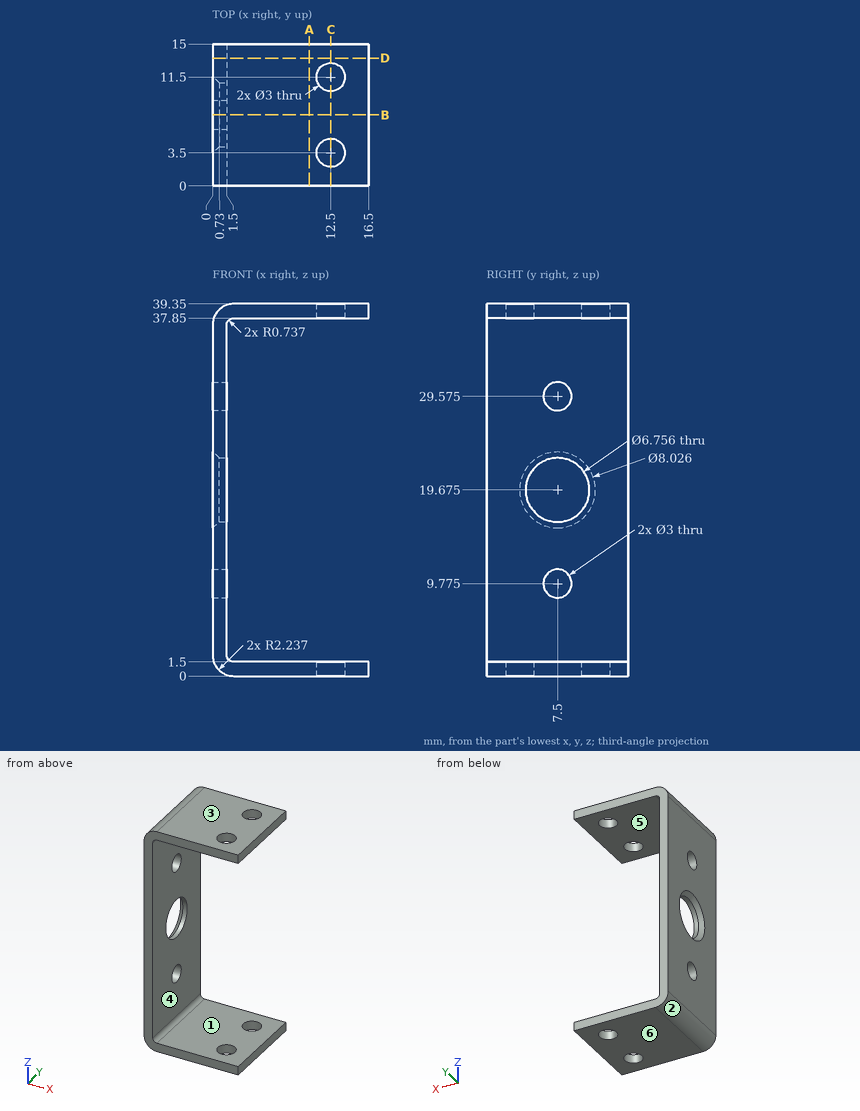
Design review of the part shown in the three views and the two pictorial views. Dimensions are in mm from the part's minimum x, y and z. A direction names the side the tool comes from. Round coordinates to 2 decimals unless told otherwise and drop trailing zeros. Write each loop counter-clockwise with the first axis right and the second up, starting at its lowest first coordinate (ties: lowest second). Pieces come first, ordered by that corner, then holes.
Item 1: Consider section C-C on x = 12.5. Give the boundary of the cut face in (y, z).
Item 2: For pin 1 Ø6 at (y, z) = (9.5, 13.5) entering from +X, flat-tipped, find the tip position at first contact; note if it passes through.
Item 3: Wall thickness on L1, parallel to Y at x = 12.5, z = 39; L2, parallel to Z at x = 4.25, y = 2: over which ranges is each line inside the solid? List them lowest first.
Item 4: Consider section D-D on y = 13.5. Give the boundary of the cut face in (x, z), and give its area (3 significant figures).
Item 5: For the marked faces 1 and 2, list the 3-axis set-ups (+Z, -Z, +X, -X, +Y, -Y) from which the entire face can be reached by the end or side of a thin tool; tool diameter is ignored.
Item 6: Consider section A-A on x = 10.25. Give the boundary of the cut face in (y, z).
Item 7: Draft analysis for pull direction Z (two halves, no side actions). For the marked faces 3, 4, 5 and 6, state which applies: released by +Z, released by -Z, zero draft, split by the parting line, or undercut.
Item 8: Consider section B-B on y = 7.5. Count the separate pieces of the cut face and the enclosed holes in it.
Check values:
1. outline: (0, 0) - (2, 0) - (2, 1.5) - (0, 1.5) - close; (0, 37.85) - (2, 37.85) - (2, 39.35) - (0, 39.35) - close; (5, 0) - (10, 0) - (10, 1.5) - (5, 1.5) - close; (5, 37.85) - (10, 37.85) - (10, 39.35) - (5, 39.35) - close; (13, 0) - (15, 0) - (15, 1.5) - (13, 1.5) - close; (13, 37.85) - (15, 37.85) - (15, 39.35) - (13, 39.35) - close
2. pin 1: stops at x = 1.5
3. L1: y = 0 to 2, 5 to 10, 13 to 15
3. L2: z = 0 to 1.5, 37.85 to 39.35
4. outline: (0, 2.24) arc R2.24 ccw to (2.24, 0) - (16.5, 0) - (16.5, 1.5) - (2.24, 1.5) arc R0.74 cw to (1.5, 2.24) - (1.5, 37.11) arc R0.74 cw to (2.24, 37.85) - (16.5, 37.85) - (16.5, 39.35) - (2.24, 39.35) arc R2.24 ccw to (0, 37.11) - close
4. area: 102 mm2
5. face 1: +X, +Y, -Y
5. face 2: -Z, -X, +Y, -Y
6. outline: (0, 0) - (15, 0) - (15, 1.5) - (0, 1.5) - close; (0, 37.85) - (15, 37.85) - (15, 39.35) - (0, 39.35) - close
7. face 3: released by +Z
7. face 4: undercut
7. face 5: undercut
7. face 6: released by -Z
8. separate pieces: 4
8. enclosed holes: 0
